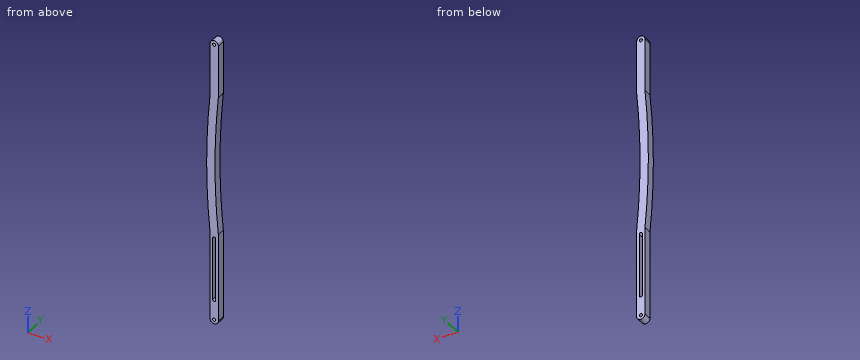
Autodesk Inventor part; units mm, degrees
ref_plane "XZ Plane" through (0, 0, 0) normal (0, 1, 0) x (-1, 0, 0)
ref_plane "XY Plane" through (0, 0, 0) normal (0, 0, 1) x (1, 0, 0)
sketch "Sketch1" plane through (0, 0, 0) normal (0, 1, 0) x (-1, 0, 0)
  line L0 (0, 0) -> (0, -270.69) construction
  line L1 (-4, 0) -> (-4, -270.69)
  line L2 (4, -270.69) -> (4, 0)
  arc A0 (4, 0) -> (-4, 0) centre (0, 0) ccw
  arc A1 (-4, -270.69) -> (4, -270.69) centre (0, -270.69) ccw
  circle A2 centre (0, 0) radius 1.5
  circle A3 centre (0, -270.69) radius 1.5
  line L3 (0, -251.19) -> (0, -190.69) construction
  line L4 (1.5, -251.19) -> (1.5, -190.69)
  line L5 (-1.5, -190.69) -> (-1.5, -251.19)
  arc A4 (-1.5, -251.19) -> (1.5, -251.19) centre (0, -251.19) ccw
  arc A5 (1.5, -190.69) -> (-1.5, -190.69) centre (0, -190.69) ccw
  arc A6 (-4, -185.69) -> (-4, -50.69) centre (-700.7379, -118.19) ccw
  arc A7 (4, -185.69) -> (4, -50.69) centre (-692.7379, -118.19) ccw
  point P0 (0, -135.345)
  point P1 (0, -220.94)
  dimension "d0" = 270.69
  dimension "d1" = 8
  dimension "d2" = 3
  dimension "d3" = 3
  dimension "d10" = 3
  dimension "d11" = 19.5
  dimension "d12" = 80
  dimension "d13" = 85
  dimension "d14" = 220
  dimension "d15" = 700
  dimension "d16" = 700
extrude "Extrusion1" add sketch "Sketch1" along normal blind 8 contours A0 L2 A1 L1 A6 | A7 L2
sketch "Sketch2" plane through (0, 0, 0) normal (0, -1, 0) x (1, 0, 0)
  line L0 (4, 0) -> (4, -50.69)
  arc A0 (4, 0) -> (-4, 0) centre (0, 0) ccw
  line L1 (-4, -50.69) -> (-4, 0)
  arc A1 (-4, -50.69) -> (-4, -185.69) centre (692.7379, -118.19) ccw
  line L2 (-4, -270.69) -> (-4, -185.69)
  arc A2 (-4, -270.69) -> (4, -270.69) centre (0, -270.69) ccw
  line L3 (4, -185.69) -> (4, -270.69)
  arc A3 (4, -50.69) -> (4, -185.69) centre (700.7379, -118.19) ccw
  circle A4 centre (0, 0) radius 1.5
  circle A5 centre (0, -270.69) radius 1.5
  arc A6 (-1.5, -251.19) -> (1.5, -251.19) centre (0, -251.19) ccw
  line L4 (-1.5, -190.69) -> (-1.5, -251.19)
  arc A7 (1.5, -190.69) -> (-1.5, -190.69) centre (0, -190.69) ccw
  line L5 (1.5, -251.19) -> (1.5, -190.69)
Model file for the job. Use its own axes, mm. Coordinates: 2 decimals unless noted, no trailing zeros. Order: outer loops, then holes, each group sorted by start corner. A loop starts at its lowest first (then second) coordinate and runs counter-clockwise, first axis right, second up. Notation, with made-up numbers: (72.5, 79) -> (102.5, 79) arc R13 cw to (102.5, 92) -> close; hole circle Ø3 at (13.25, 38.5). An arc over 180 degrees is marked (long way). Return JSON: item names as keys, results as strings. Group by question number.
Item 1: Saw through at B-B on y = 6. Write the cut outline in (x, z).
Item 2: Flat gauge pins, fed straight in: P1, Ø1, axis at x = 1.5, y = 4.5, coming from the -Z side; P2, Ø2.5, axis at y = 3, z = -246, coming from the -X side. Where does each tip first touch, or does it go through?
Item 3: Wall check: line 1 along Z through (x, y) = (0, 2); line 2 along X through (y, z) = (4, -270.69); line 3 along Z through (x, y) = (-1, 4.5). Give the ranges that are in metal, low to high. Write a range as [from, to].
Item 4: Saw through at A-A on z = -240. Write the cut outline in (x, y).
Item 5: Saw through at C-C on z = -182. Write the cut outline in (x, y), then the cut area to 3 significant figures.
Values found:
{
 "1": {"outline": "(-4, -270.69) arc R4 ccw to (4, -270.69) -> (4, -185.69) arc R700 cw to (4, -50.69) -> (4, 0) arc R4 ccw to (-4, 0) -> (-4, -50.69) arc R700 ccw to (-4, -185.69) -> close; hole circle Ø3 at (0, -270.69); hole (-1.5, -251.19) arc R1.5 ccw to (1.5, -251.19) -> (1.5, -190.69) arc R1.5 ccw to (-1.5, -190.69) -> close; hole circle Ø3 at (0, 0)"},
 "2": {"P1": "stops at z = -274.56", "P2": "stops at x = -4"},
 "3": {"line 1": "z = [-274.69, -272.19], [-269.19, -252.69], [-189.19, -1.5], [1.5, 4]", "line 2": "x = [-4, -1.5], [1.5, 4]", "line 3": "z = [-274.56, -271.81], [-269.57, -252.31], [-189.57, -1.12], [1.12, 3.87]"},
 "4": {"outline": "(-4, 0) -> (-1.5, 0) -> (-1.5, 8) -> (-4, 8) -> close; (1.5, 0) -> (4, 0) -> (4, 8) -> (1.5, 8) -> close"},
 "5": {"outline": "(-4.35, 0) -> (3.65, 0) -> (3.65, 8) -> (-4.35, 8) -> close", "area": "64.0 mm2"}
}
